Can you work these out from the model? Positions are in its coordinate system, mm. A direction names the side the tool comes from. Coordinates: 2 decimals unless noted, no trailing zeros. Order: outer loops, then holes, each group sorted by start corner. A loop starts at its lowest first (then second) coordinate and runs counter-clockwise, first axis right, second up.
```python
from build123d import *

# Parameters (mm, degrees)
SKETCH1_R          = 150
SKETCH1_R_2        = 100
EXTRUDE1_DEPTH     = 20
SKETCH2_R          = 17.5
CUT_EXTRUDE1_DEPTH = 10


with BuildPart() as part:
    # Sketch1 → Extrude1 (new body)
    with BuildSketch(Plane(origin=(0, 0, 0), x_dir=(1, 0, 0), z_dir=(0, 1, 0))):
        with Locations(Location((0, 0, 0), (0, 0, 270))):
            Circle(SKETCH1_R)
        with Locations(Location((0, 0, 0), (0, 0, 270))):
            Circle(SKETCH1_R_2, mode=Mode.SUBTRACT)
    extrude(amount=-EXTRUDE1_DEPTH)

    # Sketch2 → Cut-Extrude1 (cut)
    with BuildSketch(Plane(origin=(0, 0, 0), x_dir=(1, 0, 0), z_dir=(0, 1, 0))):
        with Locations(Location((0, 125, 0), (0, 0, 270))):
            Circle(SKETCH2_R)
        with Locations(Location((42.752517916, 117.461577598, 0), (0, 0, 270))):
            Circle(SKETCH2_R)
        with Locations(Location((108.253175473, -62.5, 0), (0, 0, 270))):
            Circle(SKETCH2_R)
        with Locations(Location((80.348451211, -95.75555539, 0), (0, 0, 270))):
            Circle(SKETCH2_R)
        with Locations(Location((-108.253175473, -62.5, 0), (0, 0, 270))):
            Circle(SKETCH2_R)
        with Locations(Location((-123.100969127, -21.706022208, 0), (0, 0, 270))):
            Circle(SKETCH2_R)
    extrude(amount=-CUT_EXTRUDE1_DEPTH, mode=Mode.SUBTRACT)


solid = part.part
```
1. Imagine slicing it at B-B on x = 38.5. Please give me the cut outline in (y, z) (3 decimals), then the cut area to 3 significant figures.
Completed:
outline: (-20, -144.975) - (0, -144.975) - (0, -134.437) - (-10, -134.437) - (-10, -100.486) - (0, -100.486) - (0, -92.292) - (-20, -92.292) - close; (-20, 92.292) - (0, 92.292) - (0, 144.975) - (-20, 144.975) - close
area: 1,770 mm2
2. I'm going to push flat-ended pins straight in: pin 1 (21 mm diameter, centred on x = -123.1, z = 21.71, fed in from +Y); pin 2 (8 mm diameter, centred on x = -101.5, y = -3, fed in from -Z); pin 3 (3 mm diameter, centred on y = -8, z = 87.5, fed in from -X); pin 4 (8 mm diameter, centred on x = 2.5, y = -15.5, fed in from -Z). Where does each tip first touch, or does it pass through?
Completed:
pin 1: stops at y = -10
pin 2: stops at z = -113.99
pin 3: stops at x = -122.9
pin 4: stops at z = -150
3. Thinking about a two-plate mould opening in X: for faces 1 (the cylindrical face through (-91.273, -9.86, -119.035)), 2 (the flat face through (-108, -10, 62)), 3 (the flat face through (-98, -20, 31)), which applies, pulls with the +X half, pulls with the -X half, needs draft (parallel to the pull), parting line crosses it, or undercut?
Completed:
face 1: parting line crosses it
face 2: undercut
face 3: needs draft
4. Imagine slicing it at D-D on x = -112.5. Please give me the cut outline in (y, z), then the cut area to 3 significant figures.
Completed:
outline: (-20, -99.22) - (0, -99.22) - (0, 7.78) - (-10, 7.78) - (-10, 35.63) - (0, 35.63) - (0, 45.52) - (-10, 45.52) - (-10, 79.48) - (0, 79.48) - (0, 99.22) - (-20, 99.22) - close
area: 3,350 mm2
5. Please list where these lines run through material, in increasing order: probe 1 along X at (y, z) = (-7.75, -129); probe 2 along Z at (x, y) = (-10, -9.25); probe 3 along X at (y, z) = (-1.5, 16).
Completed:
probe 1: x = -76.54 to -17.04, 17.04 to 29.6, 55.91 to 76.54
probe 2: z = -149.67 to -139.36, -110.64 to -99.5, 99.5 to 149.67
probe 3: x = -149.14 to -139.64, -106.56 to -98.71, 98.71 to 149.14
6. Imagine slicing it at A-A on z = 62.5. Please give me the cut outline in (x, y).
Completed:
outline: (-136.36, -20) - (-78.06, -20) - (-78.06, 0) - (-90.75, 0) - (-90.75, -10) - (-125.75, -10) - (-125.75, 0) - (-136.36, 0) - close; (78.06, -20) - (136.36, -20) - (136.36, 0) - (125.75, 0) - (125.75, -10) - (90.75, -10) - (90.75, 0) - (78.06, 0) - close
7. Imagine slicing it at C-C on y = -14.75. Please give me the cut outline in (x, z).
Completed:
outline: circle Ø300 at (0, 0); hole circle Ø200 at (0, 0)
8. On a 3-axis mill with a long thin cutter (end or side, diameter ignored), from which of +Z, -Z, +X, -X, +Y, -Y can I reach the whole of each face in a straight line? I mean faces 4 (the flat face through (-98, 0, 31)), 5 (the flat face through (108, -10, 62)). Say none if no direction works.
Completed:
face 4: +Z, -Z, +X, -X, +Y
face 5: +Y
